Verification items for the finished model (mm, model axes). A direction names the side the tool comes from. Give positions to 0.01 mm unless a question says otherwise; leave off trailing zeros. Order: outer loops, then holes, each group sorted by start corner. A loop starts at its lowest first (then second) coordinate and runs counter-clockwise, first axis right, second up.
(1) Access from +Z, -Z, +X, -X, +Y, -Y to the whole of each face (thin tool, end or side, straight path). Record for faces 5 (the face through (-21, -23, 11)), 6 (the face through (17, -23, 62)), 7 (the face through (7, -39, 20)), 8 (the face through (-27.5, -17, 5)).
(2) Sectioned sample at B-B on z = 122. Record the cut outline in (x, y).
(3) Scan lines: L1, parallel to X at y = -23.7, z = 88.29 (3 decimals); L2, parallel to X at y = -23.4, z = 140; L3, parallel to Y at x = 26, z = 0.9. Record each from-to range of solid material in increasing order.
(4) Mould release check, pull along Z, two halves, no side actions. Record for faces 1 (the face through (2, -21.5, 66)), 2 (the face through (-6, -23, 92)), 3 (the face through (21, -23, 11)), 4 (the face through (5.52, -51.49, 27.15)): pulls with the +Z half, pulls with the -Z half, needs draft (parallel to the pull), parting line crosses it, or undercut.
(5) Gauge pin test, flat ends, axial feed: pin 1 (5 mm diameter, centred on x = 26, y = 0, fed in from +Z); pin 2 (5 mm diameter, centred on x = 17, z = 140, fed in from +Y); pin 3 (2.5 mm diameter, centred on x = -9, y = -33, fed in from +Z); pin 4 (3.5 mm diameter, centred on x = -26, y = 0, fed in from -Z). Record the tip position at first contact, or that the pin passes through.
(6) Sectioned sample at C-C on z = 54.5. Record the cut outline in (x, y) (3 decimals).
(7) Sectioned sample at A-A on z = 74. Record the cut outline in (x, y) (3 decimals), plus the area to 3 significant figures.
```python
from build123d import *

# Parameters (mm, degrees)
SKETCH_1_R           = 2.1
EXTRUDE_1_DEPTH      = 3
SKETCH_2_W           = 60
SKETCH_2_H           = 3
EXTRUDE_2_DEPTH      = 80
SKETCH_3_W           = 60
SKETCH_3_H           = 3
EXTRUDE_3_DEPTH      = 60
SKETCH_4_R           = 2.1
SKETCH_4_W           = 22
SKETCH_4_H           = 42
CUT_EXTRUDE_1_DEPTH  = 149.321441471
SKETCH_5_W           = 14
SKETCH_5_H           = 20
EXTRUDE_4_DEPTH      = 30
SKETCH_6_W           = 8
SKETCH_6_H           = 30
CUT_EXTRUDE_2_DEPTH  = 129.993216876
SKETCH_7_R           = 1.05
CUT_EXTRUDE_3_DEPTH  = 158.442846773
SKETCH_8_W           = 2
SKETCH_8_H           = 7
CUT_EXTRUDE_4_DEPTH  = 150.793190766
SKETCH_9_W           = 12
SKETCH_9_H           = 132
CUT_EXTRUDE_5_DEPTH  = 150.793190766
SKETCH_12_W          = 4
SKETCH_12_H          = 6
EXTRUDE_5_DEPTH      = 3
SKETCH_13_R          = 1.6
CUT_EXTRUDE_8_DEPTH  = 150.793190766
RIB_25_REACH         = 164.958
SKETCH_19_WALL_W     = 343.147179466
SKETCH_19_WALL_H     = 3
RIB_30_REACH         = 164.958
SKETCH_20_WALL_W     = 343.147179466
SKETCH_20_WALL_H     = 3
RIB_38_REACH         = 139.838
SKETCH_21_WALL_W     = 292.907080128
SKETCH_21_WALL_H     = 3
RIB_39_REACH         = 139.838
SKETCH_22_WALL_W     = 292.907080128
SKETCH_22_WALL_H     = 3
CUT_EXTRUDE_9_DEPTH  = 150.793190766
SKETCH_24_W          = 6
SKETCH_24_H          = 51
CUT_EXTRUDE_10_DEPTH = 150.793190766
FILLET_1_R           = 5
FILLET_2_R           = 2
FILLET_3_R           = 10


with BuildPart() as part:
    # 草图1 → 凸台-拉伸1 (new body)
    with BuildSketch(Plane.XY):
        with BuildLine():
            Line((-22, 0), (-22, -21.5))
            Line((-22, -21.5), (22, -21.5))
            Line((22, -21.5), (22, 0))
            ThreePointArc((22, 0), (26, 4), (30, 0))
            Line((30, 0), (30, -24.5))
            Line((30, -24.5), (-30, -24.5))
            Line((-30, -24.5), (-30, 0))
            ThreePointArc((-30, 0), (-26, 4), (-22, 0))
        make_face()
        with Locations((-26, 0)):
            Circle(SKETCH_1_R, mode=Mode.SUBTRACT)
        with Locations((26, 0)):
            Circle(SKETCH_1_R, mode=Mode.SUBTRACT)
    extrude(amount=EXTRUDE_1_DEPTH)

    # 草图2 → 凸台-拉伸2 (add)
    with BuildSketch(Plane.XY.offset(3)):
        with Locations((0, -23)):
            Rectangle(SKETCH_2_W, SKETCH_2_H)
    extrude(amount=EXTRUDE_2_DEPTH)

    # 草图3 → 凸台-拉伸3 (add)
    with BuildSketch(Plane.XY.offset(83)):
        with Locations((0, -23)):
            Rectangle(SKETCH_3_W, SKETCH_3_H)
    extrude(amount=EXTRUDE_3_DEPTH)

    # 草图4 → 切除-拉伸1 (cut, through all)
    with BuildSketch(Plane(origin=(0, -21.5, 0), x_dir=(1, 0, 0), z_dir=(0, 1, 0))):
        with Locations(Location((-4.925, -88.29, 0), (0, 0, 270))):
            Circle(SKETCH_4_R)
        with Locations(Location((4.925, -88.29, 0), (0, 0, 270))):
            Circle(SKETCH_4_R)
        with Locations(Location((-4.925, -137.71, 0), (0, 0, 270))):
            Circle(SKETCH_4_R)
        with Locations(Location((4.925, -137.71, 0), (0, 0, 270))):
            Circle(SKETCH_4_R)
        with Locations((0, -113)):
            Rectangle(SKETCH_4_W, SKETCH_4_H)
    extrude(amount=-CUT_EXTRUDE_1_DEPTH, mode=Mode.SUBTRACT)

    # 草图5 → 凸台-拉伸4 (add)
    with BuildSketch(Plane.XZ.offset(24.5)):
        with Locations((0, 20)):
            Rectangle(SKETCH_5_W, SKETCH_5_H)
    extrude(amount=EXTRUDE_4_DEPTH)

    # 草图6 → 切除-拉伸2 (cut, through all)
    with BuildSketch(Plane.XY.offset(30)):
        with Locations((0, -39.5)):
            Rectangle(SKETCH_6_W, SKETCH_6_H)
    extrude(amount=-CUT_EXTRUDE_2_DEPTH, mode=Mode.SUBTRACT)

    # 草图7 → 切除-拉伸3 (cut, through all)
    with BuildSketch(Plane(origin=(7, 0, 0), x_dir=(0, 0, -1), z_dir=(1, 0, 0))):
        with Locations((-20, -46.5)):
            Circle(SKETCH_7_R)
    extrude(amount=-CUT_EXTRUDE_3_DEPTH, mode=Mode.SUBTRACT)

    # 草图8 → 切除-拉伸4 (cut, through all)
    with BuildSketch(Plane(origin=(0, -21.5, 0), x_dir=(1, 0, 0), z_dir=(0, 1, 0))):
        with Locations((0, -88.5)):
            Rectangle(SKETCH_8_W, SKETCH_8_H)
        with Locations((0, -137.5)):
            Rectangle(SKETCH_8_W, SKETCH_8_H)
    extrude(amount=-CUT_EXTRUDE_4_DEPTH, mode=Mode.SUBTRACT)

    # 草图9 → 切除-拉伸5 (cut, through all)
    with BuildSketch(Plane(origin=(0, -21.5, 0), x_dir=(1, 0, 0), z_dir=(0, 1, 0))):
        with Locations((24, -77)):
            Rectangle(SKETCH_9_W, SKETCH_9_H)
        with Locations((-24, -77)):
            Rectangle(SKETCH_9_W, SKETCH_9_H)
    extrude(amount=-CUT_EXTRUDE_5_DEPTH, mode=Mode.SUBTRACT)

    # 草图12 → 凸台-拉伸5 (add)
    with BuildSketch(Plane(origin=(0, -21.5, 0), x_dir=(1, 0, 0), z_dir=(0, 1, 0))):
        with Locations((20, -140)):
            Rectangle(SKETCH_12_W, SKETCH_12_H)
        with Locations((-20, -140)):
            Rectangle(SKETCH_12_W, SKETCH_12_H)
        with Locations((-20, -65)):
            Rectangle(SKETCH_12_W, SKETCH_12_H)
        with Locations((20, -65)):
            Rectangle(SKETCH_12_W, SKETCH_12_H)
    extrude(amount=-EXTRUDE_5_DEPTH)

    # 草图13 → 切除-拉伸8 (cut, through all)
    with BuildSketch(Plane(origin=(0, -21.5, 0), x_dir=(1, 0, 0), z_dir=(0, 1, 0))):
        with Locations(Location((-17, -140, 0), (0, 0, 270))):
            Circle(SKETCH_13_R)
        with Locations(Location((17, -140, 0), (0, 0, 270))):
            Circle(SKETCH_13_R)
        with Locations(Location((-17, -65, 0), (0, 0, 270))):
            Circle(SKETCH_13_R)
        with Locations(Location((17, -65, 0), (0, 0, 270))):
            Circle(SKETCH_13_R)
    extrude(amount=-CUT_EXTRUDE_8_DEPTH, mode=Mode.SUBTRACT)

    # 草图19 wall → 筋25 (add, up to next)
    with BuildSketch(Plane(origin=(-26, -14.5, 6), x_dir=(0, -0.919145030018, 0.393919298579), z_dir=(0, 0.393919298579, 0.919145030018)), mode=Mode.PRIVATE) as rib_25_sk1:
        Rectangle(SKETCH_19_WALL_W, SKETCH_19_WALL_H)
    rib_25_tool1 = extrude(rib_25_sk1.sketch, amount=-RIB_25_REACH, mode=Mode.PRIVATE) - part.part
    add(rib_25_tool1.solids().sort_by_distance((-26, -14.5, 6))[0])

    # 草图20 wall → 筋30 (add, up to next)
    with BuildSketch(Plane(origin=(26, -14.5, 6), x_dir=(0, -0.919145030018, 0.393919298579), z_dir=(0, -0.393919298579, -0.919145030018)), mode=Mode.PRIVATE) as rib_30_sk1:
        Rectangle(SKETCH_20_WALL_W, SKETCH_20_WALL_H)
    rib_30_tool1 = extrude(rib_30_sk1.sketch, amount=RIB_30_REACH, mode=Mode.PRIVATE) - part.part
    add(rib_30_tool1.solids().sort_by_distance((26, -14.5, 6))[0])

    # 草图21 wall → 筋38 (add, up to next)
    with BuildSketch(Plane(origin=(-10, -31.5, 20), x_dir=(0.393919298579, -0.919145030018, 0), z_dir=(0.919145030018, 0.393919298579, 0)), mode=Mode.PRIVATE) as rib_38_sk1:
        Rectangle(SKETCH_21_WALL_W, SKETCH_21_WALL_H)
    rib_38_tool1 = extrude(rib_38_sk1.sketch, amount=RIB_38_REACH, mode=Mode.PRIVATE) - part.part
    add(rib_38_tool1.solids().sort_by_distance((-10, -31.5, 20))[0])

    # 草图22 wall → 筋39 (add, up to next)
    with BuildSketch(Plane(origin=(10, -31.5, 20), x_dir=(-0.393919298579, -0.919145030018, 0), z_dir=(0.919145030018, -0.393919298579, 0)), mode=Mode.PRIVATE) as rib_39_sk1:
        Rectangle(SKETCH_22_WALL_W, SKETCH_22_WALL_H)
    rib_39_tool1 = extrude(rib_39_sk1.sketch, amount=-RIB_39_REACH, mode=Mode.PRIVATE) - part.part
    add(rib_39_tool1.solids().sort_by_distance((10, -31.5, 20))[0])

    # 草图23 → 切除-拉伸9 (cut, through all)
    with BuildSketch(Plane(origin=(0, -21.5, 0), x_dir=(1, 0, 0), z_dir=(0, 1, 0))):
        with BuildLine():
            Line((-5.875, -37.143702513), (-5.875, -82.143702513))
            ThreePointArc((-5.875, -82.143702513), (-7, -83.268702513), (-8.125, -82.143702513))
            Line((-8.125, -82.143702513), (-8.125, -37.143702513))
            ThreePointArc((-8.125, -37.143702513), (-7, -36.018702513), (-5.875, -37.143702513))
        make_face()
        with BuildLine():
            Line((8.125, -37.143702513), (8.125, -82.143702513))
            ThreePointArc((8.125, -82.143702513), (7, -83.268702513), (5.875, -82.143702513))
            Line((5.875, -82.143702513), (5.875, -37.143702513))
            ThreePointArc((5.875, -37.143702513), (7, -36.018702513), (8.125, -37.143702513))
        make_face()
    extrude(amount=-CUT_EXTRUDE_9_DEPTH, mode=Mode.SUBTRACT)

    # 草图24 → 切除-拉伸10 (cut, through all)
    with BuildSketch(Plane(origin=(0, -21.5, 0), x_dir=(1, 0, 0), z_dir=(0, 1, 0))):
        with Locations((-15, -36.5)):
            Rectangle(SKETCH_24_W, SKETCH_24_H)
        with Locations((15, -36.5)):
            Rectangle(SKETCH_24_W, SKETCH_24_H)
    extrude(amount=-CUT_EXTRUDE_10_DEPTH, mode=Mode.SUBTRACT)

    # 圆角1
    fillet_1_edges = [part.edges().sort_by_distance(p)[0] for p in [
        (30, -23, 11),
        (-30, -23, 11),
        (-12, -23, 11),
        (12, -23, 11),
    ]]
    fillet(fillet_1_edges, radius=FILLET_1_R)

    # 圆角2
    fillet_2_edges = [part.edges().sort_by_distance(p)[0] for p in [
        (18, -23, 137),
        (22, -23, 137),
        (22, -23, 143),
        (-22, -23, 143),
        (-22, -23, 137),
        (-18, -23, 137),
        (-18, -23, 68),
        (18, -23, 68),
        (22, -23, 68),
        (22, -23, 62),
        (12, -23, 62),
        (-22, -23, 62),
        (-12, -23, 62),
        (-22, -23, 68),
    ]]
    fillet(fillet_2_edges, radius=FILLET_2_R - 0.0001)  # a hair under: the kernel refuses the full size

    # 圆角3
    fillet_3_edges = [part.edges().sort_by_distance(p)[0] for p in [
        (5.5, -54.5, 10),
        (-5.5, -54.5, 10),
        (-5.5, -54.5, 30),
        (5.5, -54.5, 30),
    ]]
    fillet(fillet_3_edges, radius=FILLET_3_R - 0.0001)  # a hair under: the kernel refuses the full size


solid = part.part
```
Ans:
1. face 5: -X, +Y, -Y
1. face 6: +X, +Y, -Y
1. face 7: +X, -Y
1. face 8: +Z, -X, +Y
2. outline: (-18, -24.5) - (-11, -24.5) - (-11, -21.5) - (-18, -21.5) - close; (11, -24.5) - (18, -24.5) - (18, -21.5) - (11, -21.5) - close
3. L1: x = -18 to -7.025, -2.825 to -1, 1 to 2.825, 7.025 to 18
3. L2: x = -22 to -18.6, -15.4 to -1, 1 to 15.4, 18.6 to 22
3. L3: y = -24.5 to -2.1, 2.1 to 4
4. face 1: needs draft
4. face 2: undercut
4. face 3: undercut
4. face 4: pulls with the +Z half
5. pin 1: stops at z = 3
5. pin 2: stops at y = -21.5
5. pin 3: stops at z = 21.5
5. pin 4: passes through
6. outline: (-12, -24.5) - (-8.125, -24.5) - (-8.125, -21.5) - (-12, -21.5) - close; (-5.875, -24.5) - (5.875, -24.5) - (5.875, -21.5) - (-5.875, -21.5) - close; (8.125, -24.5) - (12, -24.5) - (12, -21.5) - (8.125, -21.5) - close
7. outline: (-18, -24.5) - (-8.125, -24.5) - (-8.125, -21.5) - (-18, -21.5) - close; (-5.875, -24.5) - (5.875, -24.5) - (5.875, -21.5) - (-5.875, -21.5) - close; (8.125, -24.5) - (18, -24.5) - (18, -21.5) - (8.125, -21.5) - close
7. area: 94.5 mm2
